Input: dimensioned drawing with shaded views. Units: mm. Origin: part minimum x, y, z. A direction names the side the tool comes from. Round coordinates to 2 decimals unless told otherwise and drop trailing zeros. Loops run counter-clockwise (first coordinate to the right, second up) from the corner with the lowest first, then second, coordinate; pieces in that order, holes last. Notation, with made-up numbers: (74, -27.5) - (102, -27.5) arc R22 ccw to (102, 11.5) - close; hole circle Ø7 at (-16, -23.5). An arc over 180 degrees is marked (long way). Answer as a JSON object with one key per item and string values. Group by question number.
Item 1: Section D-D (y = 26.5). Return the cut outline in (x, z).
Item 2: Draft query along X for the marked faces 1, 2, 3 and 4. Return one class per face: released by +X, released by -X, zero draft, split by the parting line, or undercut.
Item 3: Line query: line 1 (X direction, y = 8, z = 6.45); line 2 (Y direction, x = 7, z = 7); line 3 (X direction, y = 20, z = 9.75). Output: solid intervals per line, ascending.
Item 4: Section B-B (x = 7). Return the cut outline in (y, z), plus the area to 3 significant figures.
Item 5: Section C-C (z = 7). Return the cut outline in (x, y).
Item 6: First-contact query: pin 1 (3 mm diameter, centred on y = 15.5, z = 7, fed in from +X); pin 2 (5 mm diameter, centred on x = 10.5, z = 4, fed in from +Y); pin 3 (6 mm diameter, centred on x = 7, y = 8, fed in from -Z); pin 4 (4 mm diameter, centred on x = 7, z = 1.5, fed in from -Y). Flat tips, straight axial feed; report the tip coordinate or a pass-through.
Item 7: Section A-A (y = 8). Return the cut outline in (x, z), plus the area to 3 significant figures.
Item 8: Reachability of the marked faces 5, 6, 7, 8 and 9 from +Z, -Z, +X, -X, +Y, -Y: full face, straight path, thin tool, end or side. Return the list, or none.
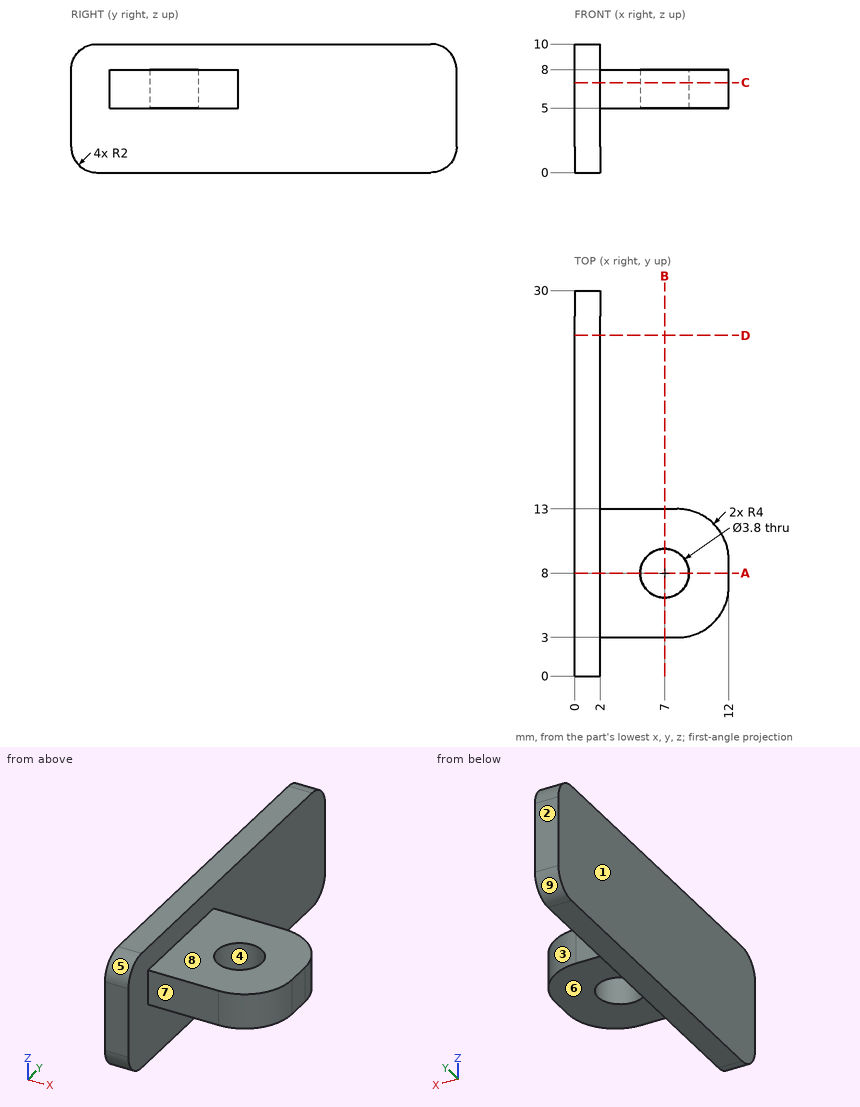
Values:
{
 "1": {"outline": "(0, 0) - (2, 0) - (2, 10) - (0, 10) - close"},
 "2": {"face 1": "released by -X", "face 2": "zero draft", "face 3": "released by +X", "face 4": "undercut"},
 "3": {"line 1": "x = 0 to 5.1, 8.9 to 12", "line 2": "y = 3 to 6.1, 9.9 to 13", "line 3": "x = 0 to 2"},
 "4": {"outline": "(3, 5) - (6.1, 5) - (6.1, 8) - (3, 8) - close; (9.9, 5) - (13, 5) - (13, 8) - (9.9, 8) - close", "area": "18.6 mm^2"},
 "5": {"outline": "(0, 0) - (2, 0) - (2, 3) - (8, 3) arc R4 ccw to (12, 7) - (12, 9) arc R4 ccw to (8, 13) - (2, 13) - (2, 30) - (0, 30) - close; hole circle Ø3.8 at (7, 8)"},
 "6": {"pin 1": "stops at x = 2", "pin 2": "stops at y = 12.99", "pin 3": "stops at z = 5", "pin 4": "passes through"},
 "7": {"outline": "(0, 0) - (2, 0) - (2, 5) - (5.1, 5) - (5.1, 8) - (2, 8) - (2, 10) - (0, 10) - close; (8.9, 5) - (12, 5) - (12, 8) - (8.9, 8) - close", "area": "38.6 mm^2"},
 "8": {"face 5": "+Z, +X, -X, -Y", "face 6": "-Z, +X, +Y, -Y", "face 7": "+Z, -Z, +X, -Y", "face 8": "+Z, +X, +Y, -Y", "face 9": "-Z, +X, -X, +Y"}
}
